Autodesk Inventor part; units mm, degrees
ref_plane "YZ Plane" through (0, 0, 0) normal (1, 0, 0) x (0, 1, 0)
ref_plane "XZ Plane" through (0, 0, 0) normal (0, 1, 0) x (-1, 0, 0)
ref_plane "XY Plane" through (0, 0, 0) normal (0, 0, 1) x (1, 0, 0)
sketch "Sketch1" plane through (0, 0, 0) normal (0, 1, 0) x (-1, 0, 0)
  line L0 (0, 0) -> (-6, 0)
  line L1 (-6, 0) -> (-6, -13)
  line L2 (-6, -13) -> (0, -13)
  line L3 (0, -13) -> (0, 0)
  dimension "d0" = 6
  dimension "d1" = 13
extrude "Extrusion1" add sketch "Sketch1" along normal blind 3.5
sketch "Sketch2" plane through (0, 3.5, 0) normal (0, 1, 0) x (1, 0, 0)
  line L0 (0, 13) -> (0, 0)
  line L1 (6, 0) -> (6, 13)
  line L2 (0, 0) -> (6, 0)
  line L3 (6, 0) -> (6, 13)
  line L4 (6, 13) -> (0, 13)
  line L5 (0, 13) -> (0, 0)
  line L6 (3, 0) -> (6.25, 0) construction
  line L7 (2, 3) -> (1.5, 3)
  line L8 (1.5, 3) -> (1, 3)
  line L9 (1.5, 3) -> (2, 3) construction
  line L10 (2, 3) -> (5, 3)
  line L11 (2, 3) -> (5, 3) construction
  line L12 (5, 3) -> (5, 10)
  line L13 (5, 10) -> (1, 10)
  line L14 (1, 10) -> (1, 3)
  line L15 (1, 3) -> (5, 3)
  line L16 (5, 3) -> (5, 10)
  line L17 (5, 10) -> (1, 10)
  line L18 (1, 10) -> (1, 3)
  dimension "d41" = 3
  dimension "d42" = 1
  dimension "d44" = 1
  dimension "d45" = 3
extrude "Extrusion3" cut sketch "Sketch2" against normal blind 0.11 contours L7 L8 L14 L13 L12 L10
sketch "Sketch3" plane through (0, 3.39, 0) normal (0, 1, 0) x (1, 0, 0)
  line L0 (1, 3) -> (1, 10)
  line L1 (1, 10) -> (5, 10)
  line L2 (5, 10) -> (5, 6)
  line L3 (5, 6) -> (1, 6)
  line L4 (1, 6) -> (1, 10)
  point P0 (0, 0)
  dimension "d20" = 4
  dimension "d21" = 4
extrude "Extrusion4" add sketch "Sketch3" along normal blind 5
sketch "Sketch4" plane through (0, 0, 0) normal (0, -1, 0) x (1, 0, 0)
  line L0 (0, 0) -> (6, 0)
  line L1 (3, 0) -> (3, -1) construction
  line L2 (3, 0) -> (4, 0) construction
  line L3 (2.875, -1.125) -> (3.125, -1.125)
  line L4 (3.125, -1.125) -> (3.125, -0.875)
  line L5 (3.125, -0.875) -> (2.875, -0.875)
  line L6 (2.875, -0.875) -> (2.875, -1.125)
  line L7 (2.875, -1.125) -> (3.125, -0.875) construction
  line L8 (3.125, -1.125) -> (2.875, -0.875) construction
  line L9 (6, -13) -> (0, -13)
  line L10 (3, -13) -> (3, -12) construction
  line L11 (3, -13) -> (4, -13) construction
  line L12 (2.875, -12.125) -> (3.125, -12.125)
  line L13 (3.125, -12.125) -> (3.125, -11.875)
  line L14 (3.125, -11.875) -> (2.875, -11.875)
  line L15 (2.875, -11.875) -> (2.875, -12.125)
  line L16 (2.875, -12.125) -> (3.125, -11.875) construction
  line L17 (3.125, -12.125) -> (2.875, -11.875) construction
  line L18 (3, -0.875) -> (3, -6.5) construction
  line L19 (3, -0.875) -> (8.625, -0.875) construction
  line L20 (2.875, -6.625) -> (3.125, -6.625)
  line L21 (3.125, -6.625) -> (3.125, -6.375)
  line L22 (3.125, -6.375) -> (2.875, -6.375)
  line L23 (2.875, -6.375) -> (2.875, -6.625)
  line L24 (2.875, -6.625) -> (3.125, -6.375) construction
  line L25 (3.125, -6.625) -> (2.875, -6.375) construction
  point P0 (3, -6.5)
  dimension "d24" = 1
  dimension "d25" = 90
  dimension "d26" = 0.25
  dimension "d27" = 0.25
  dimension "d28" = 1
  dimension "d29" = 90
  dimension "d30" = 0.25
  dimension "d31" = 0.25
  dimension "d33" = 90
  dimension "d34" = 0.25
  dimension "d35" = 0.25
  dimension "d39" = 5.5
  dimension "d40" = 5.5
extrude "Extrusion5" add sketch "Sketch4" along normal blind 7
equation "\"d41\" = d5"
equation "\"d44\" = d42"
equation "\"d45\" = d41"
equation "\"d21\" = d20"
equation "\"d24\" = d28"
properties part number "switch small"
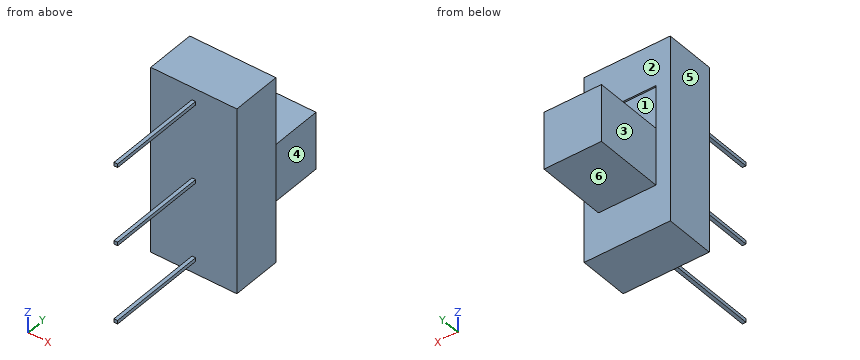
Input: part model. Units: mm. Frame: model coordinates. Face numbers are marked on the shaded views. A direction names the side the tool comes from. Give positions to 0.01 mm unless a question says otherwise; leave off trailing zeros. Loops run counter-clockwise (first coordinate to the right, second up) from the corner with the lowest first, then second, coordinate; pieces in that order, holes last. Notation, with made-up numbers: (-27.5, 65) - (-10.5, 65) arc R29 ccw to (-10.5, 103) - close; hole circle Ø5 at (43, 75). An arc over 180 degrees is marked (long way). Use CSV: the item, a comma, the result in double quotes. Start each with the question number.
Item 1: Section D-D on z = -8.75. Return loops of the section in (x, y).
Item 2: Line query: line 1 (Y direction, x = 5.7, z = -6.75); line 2 (Y direction, x = 4.9, z = -9.75); line 3 (X direction, y = 4, z = -8.5). Output: solid intervals per line, ascending.
Item 3: Reachability of the marked faces 4, 5 and 6 from +Z, -Z, +X, -X, +Y, -Y: full face, straight path, thin tool, end or side. Return the list, or none.
Item 4: Mould query, pull axis X, two halves, no side actions, for the marked faces 1, 2 and 3. Classes: pulls with the +X half, pulls with the -X half, needs draft (parallel to the pull), parting line crosses it, or undercut.
Item 5: Contact query for flat-ended pins moving along their axis: P1, Ø1, axis at x = 3, y = 6, coming from the +Z side; P2, Ø1.5, axis at x = 4, y = -5, coming from the +Z side; P3, Ø2, axis at x = 3, z = -9.5, coming from the -Y side; P4, Ø3, axis at y = 6.5, z = -8, coming from the +X side. Output: stop coordinate, or through.
Item 6: Section B-B on x = 3.5. Return loops of the section in (y, z).
Item 7: Section A-A on y = -5.75. Return loops of the section in (x, z) (3 decimals), then the cut area to 4 significant figures.
Item 8: Section C-C on z = -3.75. Return loops of the section in (x, y).
Ans:
1,outline,"(0, 0) - (6, 0) - (6, 3.5) - (5, 3.5) - (5, 8.39) - (1, 8.39) - (1, 3.5) - (0, 3.5) - close"
2,line 1,"y = 0 to 3.5"
2,line 2,"y = 0 to 8.39"
2,line 3,"x = 1 to 5"
3,face 4,"+Z, -Z, +X, +Y"
3,face 5,"+Z, -Z, -X, +Y, -Y"
3,face 6,"-Z, +X, -X, +Y"
4,face 1,"undercut"
4,face 2,"needs draft"
4,face 3,"pulls with the -X half"
5,P1,"stops at z = -6"
5,P2,"passes through"
5,P3,"stops at y = 0"
5,P4,"stops at x = 5"
6,outline,"(0, -13) - (3.5, -13) - (3.5, -10) - (8.39, -10) - (8.39, -6) - (3.39, -6) - (3.39, -3) - (3.5, -3) - (3.5, 0) - (0, 0) - close"
7,outline,"(2.875, -12.125) - (3.125, -12.125) - (3.125, -11.875) - (2.875, -11.875) - close; (2.875, -6.625) - (3.125, -6.625) - (3.125, -6.375) - (2.875, -6.375) - close; (2.875, -1.125) - (3.125, -1.125) - (3.125, -0.875) - (2.875, -0.875) - close"
7,area,"0.1875 mm2"
8,outline,"(0, 0) - (6, 0) - (6, 3.5) - (5, 3.5) - (5, 3.39) - (1, 3.39) - (1, 3.5) - (0, 3.5) - close"
